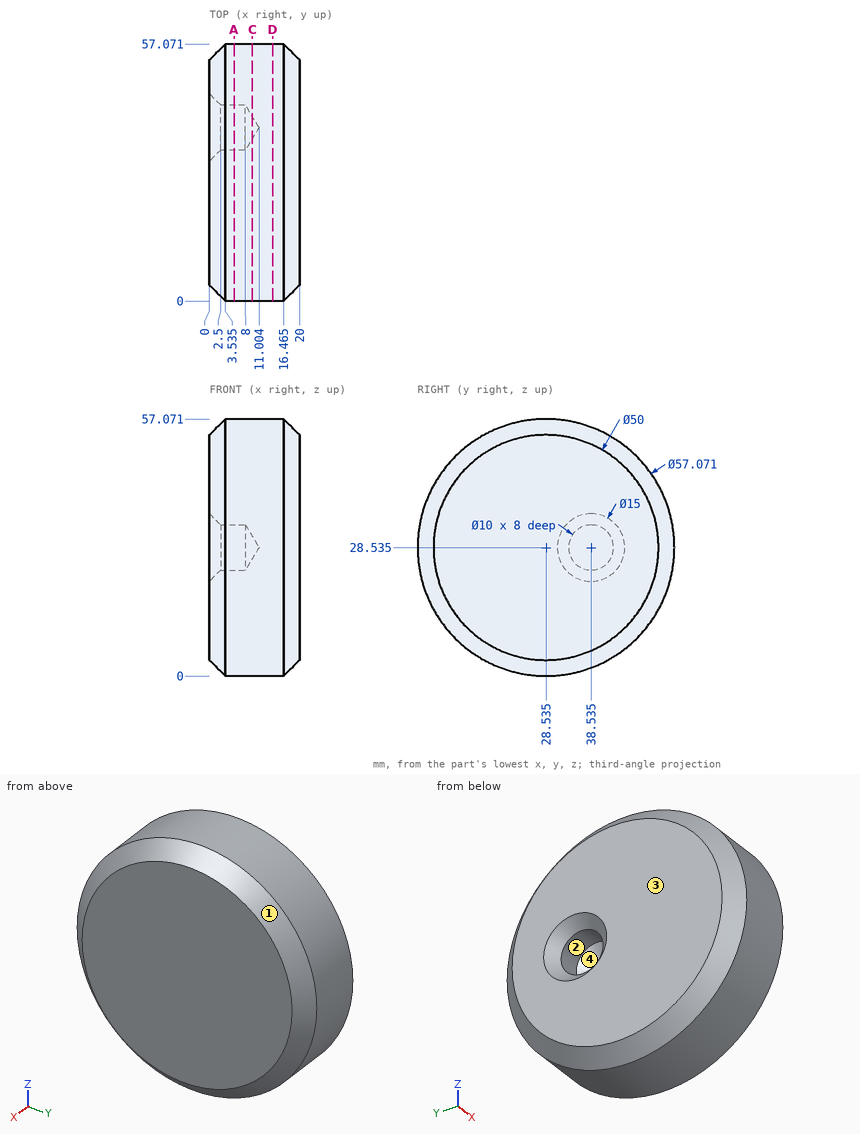
Part print with two shaded views. Sizes in mm from the minimum x, y, z corner. Round coordinates to 2 decimals unless told otherwise and drop trailing zeros. Loops run counter-clockwise (first coordinate to the right, second up) from the corner with the lowest first, then second, coordinate; pieces in that order, holes last. Notation, with made-up numbers: (49, 23) - (105, 23) arc R21 ccw to (105, 52) - close; hole circle Ø8 at (10, 29.5). An arc over 180 degrees is marked (long way). Put each result on its own line as item: value.
1. Slice it at D-D on x = 14. List the corners of the cut face in (y, z) (1 decimal).
Geometry check:
outline: circle Ø57.1 at (28.5, 28.5)
2. Slice it at C-C on x = 9.5. List the corners of the cut face in (y, z) (1 decimal).
Geometry check:
outline: circle Ø57.1 at (28.5, 28.5); hole circle Ø5 at (38.5, 28.5)
3. Pin check, flat tips, straight feed: P1, Ø4, axis at x = 10, y = 10, coming from the +Z side; P2, Ø1.5, axis at x = 13, y = 12, coming from the +Z side; P3, Ø3, axis at x = 2, y = 18.5, coming from the +Z side. Stop position of each tip, or through.
Geometry check:
P1: z = 51.79
P2: z = 52.31
P3: z = 55.3
4. Slice it at A-A on x = 5.5. List the corners of the cut face in (y, z) (1 decimal).
Geometry check:
outline: circle Ø57.1 at (28.5, 28.5); hole circle Ø10 at (38.5, 28.5)
5. Wall check: line 1 (Z direction, x = 17, y = 50) (1 decimal); line 2 (Z direction, x = 5.25, y = 31.5) (1 decimal); line 3 (Y direction, x = 2.25, z = 31) (1 decimal). Give the ranges that are in metal, low to high.
Geometry check:
line 1: 10.6 to 46.5
line 2: 0.2 to 56.9
line 3: 1.4 to 33.9, 43.2 to 55.7
6. Two-plate mould, pull along Z, no slides. Class the marked faces 1, 2, 3 and 4: released by +Z, released by -Z, zero draft, split by the parting line, or undercut.
Geometry check:
face 1: split by the parting line
face 2: undercut
face 3: zero draft
face 4: undercut
